from build123d import *
from build123d.topology import SkipClean

# Parameters (mm, degrees)
SKETCH_1_R          = 24
SKETCH_1_R_2        = 1.6
SKETCH_1_W          = 15
SKETCH_1_H          = 15
SKETCH_1_R_3        = 1.3
EXTRUDE_1_DEPTH     = 2.5
SKETCH_1_4_R        = 26
SKETCH_1_4_R_2      = 24
EXTRUDE_2_DEPTH     = 14
SKETCH_1_6_R        = 1.3
EXTRUDE_4_DEPTH     = 5
CUT_EXTRUDE_1_DEPTH = 12.1
EXTRUDE_5_DEPTH     = 6.6
SKETCH_1_11_R       = 2.3
SKETCH_1_11_R_2     = 1.3
CUT_EXTRUDE_2_DEPTH = 2.5
CUT_EXTRUDE_5_DEPTH = 5.5
EXTRUDE_6_DEPTH     = 2.5


with BuildPart() as part:
    # Sketch 1 → Extrude 1 (new body)
    with BuildSketch(Plane(origin=(0, 0, 0), x_dir=(1, 0, 0), z_dir=(0, 1, 0))):
        with Locations(Location((0, 0, 0), (0, 0, 270))):
            Circle(SKETCH_1_R)
        with BuildLine():
            ThreePointArc((-11.939965885, 14.590752164), (-11.887, 14.1), (-11.939965885, 13.609247836))
            Line((-11.939965885, 13.609247836), (-11.939965885, 14.590752164))
        make_face(mode=Mode.SUBTRACT)
        with Locations(Location((0, -15, 0), (0, 0, 270))):
            Circle(SKETCH_1_R_2, mode=Mode.SUBTRACT)
        with Locations(Location((-15, 0, 0), (0, 0, 270))):
            Circle(SKETCH_1_R_2, mode=Mode.SUBTRACT)
        Rectangle(SKETCH_1_W, SKETCH_1_H, mode=Mode.SUBTRACT)
        with Locations(Location((15, 0, 0), (0, 0, 270))):
            Circle(SKETCH_1_R_2, mode=Mode.SUBTRACT)
        with Locations(Location((0, 15, 0), (0, 0, 270))):
            Circle(SKETCH_1_R_2, mode=Mode.SUBTRACT)
        with Locations(Location((-14.187, 14.1, 0), (0, 0, 270))):
            Circle(SKETCH_1_R_3, mode=Mode.SUBTRACT)
        with Locations(Location((-20.498, 0, 0), (0, 0, 270))):
            Circle(SKETCH_1_R_3, mode=Mode.SUBTRACT)
        with Locations(Location((-14.187, -14.1, 0), (0, 0, 270))):
            Circle(SKETCH_1_R_3, mode=Mode.SUBTRACT)
        with Locations(Location((14.872, -14.097, 0), (0, 0, 270))):
            Circle(SKETCH_1_R_3, mode=Mode.SUBTRACT)
        with Locations(Location((20.498, 0, 0), (0, 0, 270))):
            Circle(SKETCH_1_R_3, mode=Mode.SUBTRACT)
        with Locations(Location((14.872, 14.097, 0), (0, 0, 270))):
            Circle(SKETCH_1_R_3, mode=Mode.SUBTRACT)
    extrude(amount=EXTRUDE_1_DEPTH)

    # Sketch 1_4 → Extrude 2 (add)
    # profile 1 of 4: a face of its own
    with SkipClean():  # the faces are left unmerged after this step: merging them gives an invalid solid
        with BuildSketch(Plane(origin=(0, 0, 0), x_dir=(1, 0, 0), z_dir=(0, 1, 0))):
            with Locations(Location((0, 0, 0), (0, 0, 270))):
                Circle(SKETCH_1_4_R)
            with Locations(Location((0, 0, 0), (0, 0, 270))):
                Circle(SKETCH_1_4_R_2, mode=Mode.SUBTRACT)
        # profile 2 of 4: a face of its own
        with BuildSketch(Plane(origin=(0, 0, 0), x_dir=(1, 0, 0), z_dir=(0, 1, 0))):
            with BuildLine():
                ThreePointArc((-5.3490301, 23.396321869), (0, 24), (5.3490301, 23.396321869))
                Line((5.3490301, 23.396321869), (5.3490301, 25.44381805))
                ThreePointArc((5.3490301, 25.44381805), (0, 26), (-5.3490301, 25.44381805))
                Line((-5.3490301, 25.44381805), (-5.3490301, 23.396321869))
            make_face()
        # profile 3 of 4: a face of its own
        with BuildSketch(Plane(origin=(0, 0, 0), x_dir=(1, 0, 0), z_dir=(0, 1, 0))):
            with BuildLine():
                ThreePointArc((-11.939965885, 20.819154994), (-8.740011031, 22.352006782), (-5.3490301, 23.396321869))
                Line((-5.3490301, 23.396321869), (-5.3490301, 25.44381805))
                ThreePointArc((-5.3490301, 25.44381805), (-25.990956519, -0.68569618), (-4, -25.690465157))
                Line((-4, -25.690465157), (-4, -23.664319132))
                ThreePointArc((-4, -23.664319132), (-6.538430116, -23.092183345), (-9, -22.248595461))
                ThreePointArc((-9, -22.248595461), (-23.944275415, -1.634525883), (-11.939965885, 20.819154994))
            make_face()
        # profile 4 of 4: a face of its own
        with BuildSketch(Plane(origin=(0, 0, 0), x_dir=(1, 0, 0), z_dir=(0, 1, 0))):
            with BuildLine():
                Line((4, -25.690465157), (4, -23.664319132))
                ThreePointArc((4, -23.664319132), (0, -24), (-4, -23.664319132))
                Line((-4, -23.664319132), (-4, -25.690465157))
                ThreePointArc((-4, -25.690465157), (0, -26), (4, -25.690465157))
            make_face()
        extrude(amount=EXTRUDE_2_DEPTH)

    # Sketch 1_6 → Extrude 4 (add)
    # profile 1 of 2: a face of its own
    with SkipClean():  # the faces are left unmerged after this step: merging them gives an invalid solid
        with BuildSketch(Plane(origin=(0, 0, 0), x_dir=(1, 0, 0), z_dir=(0, 1, 0))):
            with BuildLine():
                Line((12.327725044, 20.59192063), (12.327725044, 12.355677376))
                ThreePointArc((12.327725044, 12.355677376), (17.325666659, -2.111123633), (9, -14.954449778))
                Line((9, -14.954449778), (9, -22.248595461))
                ThreePointArc((9, -22.248595461), (23.927921319, -1.858650415), (12.327725044, 20.59192063))
            make_face()
            with Locations(Location((14.872, -14.097, 0), (0, 0, 270))):
                Circle(SKETCH_1_6_R, mode=Mode.SUBTRACT)
            with Locations(Location((20.498, 0, 0), (0, 0, 270))):
                Circle(SKETCH_1_6_R, mode=Mode.SUBTRACT)
            with Locations(Location((14.872, 14.097, 0), (0, 0, 270))):
                Circle(SKETCH_1_6_R, mode=Mode.SUBTRACT)
        # profile 2 of 2: a face of its own
        with BuildSketch(Plane(origin=(0, 0, 0), x_dir=(1, 0, 0), z_dir=(0, 1, 0))):
            with BuildLine():
                Line((-9, -22.248595461), (-9, -14.954449778))
                ThreePointArc((-9, -14.954449778), (-17.356224893, -1.843102181), (-11.939965885, 12.73078092))
                Line((-11.939965885, 12.73078092), (-11.939965885, 20.819154994))
                ThreePointArc((-11.939965885, 20.819154994), (-23.944275415, -1.634525883), (-9, -22.248595461))
            make_face()
            with Locations(Location((-14.187, 14.1, 0), (0, 0, 270))):
                Circle(SKETCH_1_6_R, mode=Mode.SUBTRACT)
            with Locations(Location((-20.498, 0, 0), (0, 0, 270))):
                Circle(SKETCH_1_6_R, mode=Mode.SUBTRACT)
            with Locations(Location((-14.187, -14.1, 0), (0, 0, 270))):
                Circle(SKETCH_1_6_R, mode=Mode.SUBTRACT)
        extrude(amount=EXTRUDE_4_DEPTH)

    # Sketch 1_8 → Cut-Extrude 1 (cut)
    with SkipClean():  # the faces are left unmerged after this step: merging them gives an invalid solid
        with BuildSketch(Plane(origin=(0, 0, 0), x_dir=(1, 0, 0), z_dir=(0, 1, 0))):
            with BuildLine():
                ThreePointArc((-5.3490301, 23.396321869), (0, 24), (5.3490301, 23.396321869))
                Line((5.3490301, 23.396321869), (5.3490301, 25.44381805))
                ThreePointArc((5.3490301, 25.44381805), (0, 26), (-5.3490301, 25.44381805))
                Line((-5.3490301, 25.44381805), (-5.3490301, 23.396321869))
            make_face()
        extrude(amount=CUT_EXTRUDE_1_DEPTH, mode=Mode.SUBTRACT)

    # Sketch 1_9 → Extrude 5 (add)
    with SkipClean():  # the faces are left unmerged after this step: merging them gives an invalid solid
        with BuildSketch(Plane(origin=(0, 0, 0), x_dir=(1, 0, 0), z_dir=(0, 1, 0))):
            with BuildLine():
                ThreePointArc((-5.3490301, 23.396321869), (0, 24), (5.3490301, 23.396321869))
                Line((5.3490301, 23.396321869), (5.3490301, 25.44381805))
                ThreePointArc((5.3490301, 25.44381805), (0, 26), (-5.3490301, 25.44381805))
                Line((-5.3490301, 25.44381805), (-5.3490301, 23.396321869))
            make_face()
        extrude(amount=EXTRUDE_5_DEPTH)

    # Sketch 1_11 → Cut-Extrude 2 (cut)
    # profile 1 of 6: a face of its own
    with SkipClean():  # the faces are left unmerged after this step: merging them gives an invalid solid
        with BuildSketch(Plane(origin=(0, 0, 0), x_dir=(1, 0, 0), z_dir=(0, 1, 0))):
            with Locations(Location((14.872, -14.097, 0), (0, 0, 270))):
                Circle(SKETCH_1_11_R)
            with Locations(Location((14.872, -14.097, 0), (0, 0, 270))):
                Circle(SKETCH_1_11_R_2, mode=Mode.SUBTRACT)
        # profile 2 of 6: a face of its own
        with BuildSketch(Plane(origin=(0, 0, 0), x_dir=(1, 0, 0), z_dir=(0, 1, 0))):
            with Locations(Location((-14.187, -14.1, 0), (0, 0, 270))):
                Circle(SKETCH_1_11_R)
            with Locations(Location((-14.187, -14.1, 0), (0, 0, 270))):
                Circle(SKETCH_1_11_R_2, mode=Mode.SUBTRACT)
        # profile 3 of 6: a face of its own
        with BuildSketch(Plane(origin=(0, 0, 0), x_dir=(1, 0, 0), z_dir=(0, 1, 0))):
            with Locations(Location((-20.498, 0, 0), (0, 0, 270))):
                Circle(SKETCH_1_11_R)
            with Locations(Location((-20.498, 0, 0), (0, 0, 270))):
                Circle(SKETCH_1_11_R_2, mode=Mode.SUBTRACT)
        # profile 4 of 6: a face of its own
        with BuildSketch(Plane(origin=(0, 0, 0), x_dir=(1, 0, 0), z_dir=(0, 1, 0))):
            with BuildLine():
                ThreePointArc((-11.939965885, 14.590752164), (-16.487, 14.1), (-11.939965885, 13.609247836))
                Line((-11.939965885, 13.609247836), (-11.939965885, 14.590752164))
            make_face()
            with Locations(Location((-14.187, 14.1, 0), (0, 0, 270))):
                Circle(SKETCH_1_11_R_2, mode=Mode.SUBTRACT)
        # profile 5 of 6: a face of its own
        with BuildSketch(Plane(origin=(0, 0, 0), x_dir=(1, 0, 0), z_dir=(0, 1, 0))):
            with Locations(Location((14.872, 14.097, 0), (0, 0, 270))):
                Circle(SKETCH_1_11_R)
            with Locations(Location((14.872, 14.097, 0), (0, 0, 270))):
                Circle(SKETCH_1_11_R_2, mode=Mode.SUBTRACT)
        # profile 6 of 6: a face of its own
        with BuildSketch(Plane(origin=(0, 0, 0), x_dir=(1, 0, 0), z_dir=(0, 1, 0))):
            with Locations(Location((20.498, 0, 0), (0, 0, 270))):
                Circle(SKETCH_1_11_R)
            with Locations(Location((20.498, 0, 0), (0, 0, 270))):
                Circle(SKETCH_1_11_R_2, mode=Mode.SUBTRACT)
        extrude(amount=CUT_EXTRUDE_2_DEPTH, mode=Mode.SUBTRACT)

    # Sketch 1_12 → Cut-Extrude 5 (cut)
    with SkipClean():  # the faces are left unmerged after this step: merging them gives an invalid solid
        with BuildSketch(Plane(origin=(0, 0, 0), x_dir=(1, 0, 0), z_dir=(0, 1, 0))):
            with BuildLine():
                Line((4, -25.690465157), (4, -23.664319132))
                ThreePointArc((4, -23.664319132), (0, -24), (-4, -23.664319132))
                Line((-4, -23.664319132), (-4, -25.690465157))
                ThreePointArc((-4, -25.690465157), (0, -26), (4, -25.690465157))
            make_face()
        extrude(amount=CUT_EXTRUDE_5_DEPTH, mode=Mode.SUBTRACT)

    # Sketch 1_13 → Extrude 6 (add)
    with SkipClean():  # the faces are left unmerged after this step: merging them gives an invalid solid
        with BuildSketch(Plane(origin=(0, 0, 0), x_dir=(1, 0, 0), z_dir=(0, 1, 0))):
            with BuildLine():
                Line((4, -25.690465157), (4, -23.664319132))
                ThreePointArc((4, -23.664319132), (0, -24), (-4, -23.664319132))
                Line((-4, -23.664319132), (-4, -25.690465157))
                ThreePointArc((-4, -25.690465157), (0, -26), (4, -25.690465157))
            make_face()
        extrude(amount=EXTRUDE_6_DEPTH)


solid = part.part
The listing builds one solid part. Answer for the finished solid, in the listing's coordinates (mm). A direction names the side the tool comes from. Round coordinates to 2 decimals unless told otherwise and drop trailing zeros. Write each loop counter-clockwise with the first axis right and the second up, starting at its lowest first coordinate (ties: lowest second). Pieces come first, ordered by that corner, then holes. Notation, with made-up numbers: M -35,35.25 L -21,35.25 A21 cw -21,60.25 Z; hole C 88,72 d6. An arc over 180 degrees is marked long. Write each question's results on one line, items separated by ' | '. Start each with the question number.
Item 1: Flat-ended cylindrical pins translate along their axes: pin 1 Ø0.6 at (y, z) = (3.5, 24) entering from +X; pin 2 Ø1.6 at (y, z) = (10, -24) entering from -X; pin 3 Ø3 at (x, y) = (-18.5, 4.5) entering from +Z; pin 4 Ø2 at (x, z) = (-20.498, 0) entering from +Y. Find the tip coordinate at first contact, or state that the pin passes through.
Item 2: For a pull along X with two mould halves and no side action, classify faces 1 (the face through (0, 1, 7.5)), 2 (the face through (-23, 14, 8)) as pulls with the +X half, pulls with the -X half, needs draft (parallel to the pull), parting line crosses it, or undercut.
Item 3: Straight lines are drawn through the part: L1, parallel to Z at x = 14.5, y = 0.75; L2, parallel to Y at x = -18.5, z = -7.5; L3, parallel to X at y = 4.55, z = 14.1. For each, find the intervals that lie inside material, in ascending order. Write a range as [from, to].
Item 4: A cutting plane is placed at A-A on z = 6.5. Write down the section's boundary in (x, y).
Item 5: For faces 3 (the face through (5.349, 9, -24)), 4 (the face through (-18.218, 1.232, -0.299)), 5 (the face through (-9, 4, 19)), determine the directions among +Z, -Z, +X, -X, +Y, -Y from which every point of the face is accessible in a straight line to the end or side of a thin tool.
Item 6: A cutting plane is placed at B-B on y = 1.5. State how many separate pieces and enclosed holes the cut face has, and give its area (3 significant figures).
Item 7: A cutting plane is placed at D-D on y = 9.5. Write down the section's boundary in (x, z).
Check sheet entries:
1) pin 1: x = 10.69 | pin 2: x = -11.74 | pin 3: z = 19.67 | pin 4: through
2) face 1: undercut | face 2: needs draft
3) L1: [-21.58, -16.37], [-11.83, -1.52], [1.52, 11.83], [16.37, 21.58] | L2: [0, 5] | L3: [-21.84, -15.49], [-12.89, -10.29], [10.29, 13.57], [16.17, 21.84]
4) outline: M -25.17,0 L -7.5,0 L -7.5,2.5 L -16.2,2.5 L -16.2,5 L -23.1,5 L -23.1,14 L -25.17,14 Z; M 7.5,0 L 25.17,0 L 25.17,14 L 23.1,14 L 23.1,5 L 16.2,5 L 16.2,2.5 L 7.5,2.5 Z
5) face 3: -Z | face 4: -Y | face 5: +Y
6) separate pieces: 1 | enclosed holes: 11 | area: 1,770 mm²
7) outline: M -5.35,-25.44 L -5.35,-23.4 A24 cw long 5.35,-23.4 L 5.35,-25.44 A26 ccw long Z
